from build123d import *

# Parameters (mm, degrees)
SKETCH1_W           = 25
SKETCH1_H           = 25
BOSS_EXTRUDE1_DEPTH = 25
SKETCH2_W           = 21
SKETCH2_H           = 21
CUT_EXTRUDE1_DEPTH  = 21
FILLET1_R           = 6
FILLET2_R           = 4


with BuildPart() as part:
    # Sketch1 → Boss-Extrude1 (new body)
    with BuildSketch(Plane(origin=(0, 0, 0), x_dir=(1, 0, 0), z_dir=(0, 1, 0))):
        with Locations((12.5, -12.5)):
            Rectangle(SKETCH1_W, SKETCH1_H)
    extrude(amount=BOSS_EXTRUDE1_DEPTH)

    # Sketch2 → Cut-Extrude1 (cut)
    with BuildSketch(Plane(origin=(0, 25, 0), x_dir=(1, 0, 0), z_dir=(0, 1, 0))):
        with Locations((14.5, -14.5)):
            Rectangle(SKETCH2_W, SKETCH2_H)
    extrude(amount=-CUT_EXTRUDE1_DEPTH, mode=Mode.SUBTRACT)

    # Fillet1
    fillet1_edges = [part.edges().sort_by_distance(p)[0] for p in [
        (25, 25, 2),
        (25, 2, 25),
        (2, 25, 25),
    ]]
    fillet(fillet1_edges, radius=FILLET1_R)

    # Sketch4 → CSK for M4 Countersunk Flat Head Screw2 (revolve, cut)
    with BuildSketch(Plane(origin=(18, 18, 0), x_dir=(0, 1, 0), z_dir=(1, 0, 0))):
        Polygon((0, 0), (0, 4), (2.25, 4), (2.25, 2.45), (4.7, 0), align=None)
    revolve(axis=Axis((18, 18, -6.35), (0, 0, 1)), mode=Mode.SUBTRACT)

    # Sketch4 at point 2 (carried to point 2, square into its face) → CSK for M4 Countersunk Flat Head Scr 2 (revolve, cut)
    with BuildSketch(Plane(origin=(0, 18, 18), x_dir=(0, 1, 0), z_dir=(0, 0, -1))):
        Polygon((0, 0), (0, 4), (2.25, 4), (2.25, 2.45), (4.7, 0), align=None)
    revolve(axis=Axis((-6.35, 18, 18), (1, 0, 0)), mode=Mode.SUBTRACT)

    # Sketch4 at point 3 (carried to point 3, square into its face) → CSK for M4 Countersunk Flat Head Scr 3 (revolve, cut)
    with BuildSketch(Plane(origin=(18, 0, 18), x_dir=(0, 0, -1), z_dir=(1, 0, 0))):
        Polygon((0, 0), (0, 4), (2.25, 4), (2.25, 2.45), (4.7, 0), align=None)
    revolve(axis=Axis((18, -6.35, 18), (0, 1, 0)), mode=Mode.SUBTRACT)

    # Fillet2
    fillet2_edges = [part.edges().sort_by_distance(p)[0] for p in [
        (12.5, 0, 0),
        (0, 0, 12.5),
        (0, 12.5, 0),
    ]]
    fillet(fillet2_edges, radius=FILLET2_R)


solid = part.part
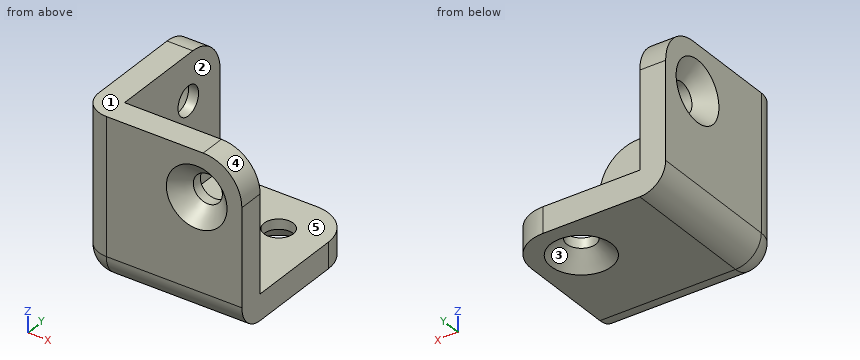
The listing builds one solid part. Answer for the finished solid, in the listing's coordinates (mm). Face numbers are marked on the shaded views. A direction names the side the tool comes from. Coordinates: 2 decimals unless noted, no trailing zeros. Write each loop counter-clockwise with the first axis right and the second up, starting at its lowest first coordinate (ties: lowest second). Pieces come first, ordered by that corner, then holes. Notation, with made-up numbers: M -28,48 L 19,48 A7 ccw 19,60 Z; hole C -14.75,-14 d4. An arc over 180 degrees is marked long. Put each result on its own line as item: value. Start each with the question number.
1. Consider line 1 (Z direction, x = 7.5, y = 16.75); line 2 (Z direction, x = 18.75, y = 1). Determine where each line is inside the solid, lowest interval first. Write a range as from..to.
2. For a pull along X with two mould halves and no side action, classify the marked faces 3, 4 and 5 as pulls with the +X half, pulls with the -X half, needs draft (parallel to the pull), parting line crosses it, or undercut.
3. A cutting plane is placed at C-C on y = 11.25. Write down the section's boundary in (x, z), then the cut area to 3 significant figures.
4. A cutting plane is placed at A-A on z = 18. Write down the section's boundary in (x, y), then the cut area to 3 significant figures.
5. Which of the six approach directions +Z, -Z, +X, -X, +Y, -Y give full straight-line access (tool end or side, diameter ignored) to the marked faces 1 and 2?
6. Flat-ended cylindrical pins translate along their axes: P1, Ø3, axis at x = 10, z = 13, coming from the +Y side; P2, Ø5, axis at y = 11.5, z = 11, coming from the +X side; P3, Ø6, axis at x = 18, y = 18, coming from the -Z side. Find the tip coordinate at first contact, or state that the pin passes through.
Resolved:
1. line 1: z = 0..4
1. line 2: z = 1.35..14.38, 21.62..25
2. face 3: undercut
2. face 4: pulls with the +X half
2. face 5: needs draft
3. outline: M 0,4 A4 ccw 4,0 L 25,0 L 25,4 L 4,4 L 4,25 L 0,25 Z
3. area: 181 mm2
4. outline: M 0,4 A4 ccw 4,0 L 13.3,0 L 15.75,2.45 L 15.75,4 L 4,4 L 4,15.75 L 2.45,15.75 L 0,13.3 Z; M 0,22.7 L 2.45,20.25 L 4,20.25 L 4,25 L 0,25 Z; M 20.25,2.45 L 22.7,0 L 25,0 L 25,4 L 20.25,4 Z
4. area: 133 mm2
5. face 1: +Z, +X, -X, +Y, -Y
5. face 2: +Z, +X, +Y
6. P1: stops at y = 4
6. P2: stops at x = 4
6. P3: stops at z = 1.7
